from build123d import *

# Parameters (mm, degrees)
F1_DEPTH = 70
F3_DEPTH = 75.001


with BuildPart() as f1:
    # F0 (on Front) → F1 (new body)
    with BuildSketch(Plane.XZ):
        Polygon((0, 75), (0, 0), (125, 0), (125, 75), (95, 75), (95, 50), (25, 50), (25, 75), align=None)
    extrude(amount=F1_DEPTH)

    # F2 (on Top) → F3 (cut, through all)
    with BuildSketch(Plane.XY):
        Polygon((0, -70), (100, -70), (100, -40), (70, -40), (70, -35), (42.5, -35), (42.5, -50), (0, -50), align=None)
    extrude(amount=F3_DEPTH, mode=Mode.SUBTRACT)


solid = f1.part
Here's how the part is built. I have some questions about the finished solid (model axes, mm). A direction names the side the tool comes from. Round coordinates to 2 decimals unless told otherwise and drop trailing zeros. Loops run counter-clockwise (first coordinate to the right, second up) from the corner with the lowest first, then second, coordinate; pieces in that order, holes last.
1. If we section it at D-D on x = 93.5: Write out the boundary of the cut face in (y, z).
Answer list:
outline: (-40, 0) - (0, 0) - (0, 50) - (-40, 50) - close
2. Which directions (+Z, -Z, +X, -X, +Y, -Y) give clear straight access to the entire face, cutting with the end or side of a thin tool? Please do faces 1 (the face through (60, -19, 50)), 2 (the face through (70, -38, 25)), 3 (the face through (22, -50, 29)).
Answer list:
face 1: +Z, +Y, -Y
face 2: +Z, -Z, -Y
face 3: +Z, -Z, -X, -Y
3. We'd pull the mould along X, two halves only. Please class faces 4 (the face through (56, -35, 25)), 5 (the face through (25, -25, 62)), 6 (the face through (62, 0, 30)), 7 (the face through (125, -35, 37)): +X half, -X half, draft (parallel to the pull), parting line (faces both ways), or undercut.
Answer list:
face 4: undercut
face 5: undercut
face 6: draft
face 7: +X half
4. If we section it at A-A on y = -48: Write out the boundary of the cut face in (x, z), plus the area to 4 significant figures.
Answer list:
outline: (0, 0) - (42.5, 0) - (42.5, 50) - (25, 50) - (25, 75) - (0, 75) - close; (100, 0) - (125, 0) - (125, 75) - (100, 75) - close
area: 4,625 mm2
5. If we section it at C-C on y = -17: Write out the boundary of the cut face in (x, z).
Answer list:
outline: (0, 0) - (125, 0) - (125, 75) - (95, 75) - (95, 50) - (25, 50) - (25, 75) - (0, 75) - close
6. If I drill on line 1 along X through (y, z) = (-46, 16.5); line 2 along X through (y, z) = (-16.5, 52); line 3 along Z through (x, y) = (28, -26), over which ranges is the centre line in solid material (lowest first)?
Answer list:
line 1: x = 0 to 42.5, 100 to 125
line 2: x = 0 to 25, 95 to 125
line 3: z = 0 to 50
7. For P1, Ø1.5, axis at y = -55.5, z = 44, coming from the -X side; P2, Ø13, axis at x = 12, z = 28, coming from the -Y side; P3, Ø15, axis at x = 54, y = -37, coming from the +Z side, each with a flat end and sliding along its axis, tell me the tip position at first contact or that it passes through.
Answer list:
P1: stops at x = 100
P2: stops at y = -50
P3: stops at z = 50
8. If we section it at B-B on z = 8: Write out the boundary of the cut face in (x, y), plus the area to 3 significant figures.
Answer list:
outline: (0, -50) - (42.5, -50) - (42.5, -35) - (70, -35) - (70, -40) - (100, -40) - (100, -70) - (125, -70) - (125, 0) - (0, 0) - close
area: 6,040 mm2
